Check sheet for the modelled part. Datum: model origin and axes. Units: mm. Round coordinates to 2 decimals unless told otherwise and drop trailing zeros. Write each loop counter-clockwise with the first axis right and the second up, starting at its lowest first coordinate (ties: lowest second). Pieces come first, ordered by that corner, then holes.
Item 1: Material ranges on line 1 along X through (y, z) = (42, 2.7); line 2 along X through (y, z) = (36, 0.9); line 3 along Y through (x, z) = (-52, 0.85), recorded low to high.
Item 2: Section check D-D, the plane z = 2.25. State how many separate pieces and enclosed holes the cut face has, plus the area to 3 significant figures.
Item 3: Section check C-C, the plane x = -11.5. Record the cut outline in (y, z), plus the area to 3 significant figures.
Item 4: Section check B-B, the plane y = 12. Record the cut outline in (x, z).
Item 5: Section check A-A, the plane y = 64. Record the cut outline in (x, z).
Item 6: Depth check by flat-ended pin: pin 1 (1.5 mm diameter, centred on y = 37, z = 1.5, fed in from +X). Enter the tip coordinate at first touch or a pass-through.
from build123d import *

# Parameters (mm, degrees)
F1_DEPTH = 3


with BuildPart() as f1:
    # F0 (on Top) → F1 (new body)
    with BuildSketch(Plane.XY):
        with BuildLine():
            Line((0, 20), (-26.666667, 20))
            ThreePointArc((-26.666667, 20), (-29.828944, 20.513167), (-32.666667, 22))
            Line((-32.666667, 22), (-30, 20))
            Line((-30, 20), (-30, 0.57191))
            ThreePointArc((-30, 0.57191), (-28.357686, 0.144014), (-26.666667, 0))
            Line((-26.666667, 0), (0, 0))
            Line((0, 0), (0, 10))
            Line((0, 10), (0, 20))
        make_face()
        with BuildLine():
            Line((26.666667, 20), (0, 20))
            Line((0, 20), (0, 10))
            Line((0, 10), (0, 0))
            Line((0, 0), (26.666667, 0))
            ThreePointArc((26.666667, 0), (28.357686, 0.144014), (30, 0.57191))
            Line((30, 0.57191), (30, 20))
            Line((30, 20), (32.666667, 22))
            ThreePointArc((32.666667, 22), (29.828944, 20.513167), (26.666667, 20))
        make_face()
        with BuildLine():
            Line((-30, 20), (-32.666667, 22))
            Line((-32.666667, 22), (-70.117305, 50.087979))
            Line((-70.117305, 50.087979), (-71.717305, 51.287979))
            Line((-71.717305, 51.287979), (-76.11797, 54.588477))
            ThreePointArc((-76.11797, 54.588477), (-78.558883, 57.226483), (-79.909473, 60.557104))
            ThreePointArc((-79.909473, 60.557104), (-104.817576, 66.113182), (-92.509473, 43.757104))
            ThreePointArc((-92.509473, 43.757104), (-88.933911, 43.393113), (-85.71797, 41.788477))
            Line((-85.71797, 41.788477), (-39.6, 7.2))
            Line((-39.6, 7.2), (-32.666667, 2))
            ThreePointArc((-32.666667, 2), (-31.387645, 1.184538), (-30, 0.57191))
            Line((-30, 0.57191), (-30, 20))
        make_face()
        Polygon((-64.226276, 29.419657), (-60.626276, 34.219657), (-56.226276, 23.419657), align=None, mode=Mode.SUBTRACT)
        Polygon((-74.7174, 37.28805), (-63.1174, 36.08805), (-66.7174, 31.28805), align=None, mode=Mode.SUBTRACT)
        Polygon((-50.3174, 31.488), (-53.9174, 26.688), (-58.3174, 37.488), align=None, mode=Mode.SUBTRACT)
        Polygon((-53.9174, 21.688), (-42.3174, 20.488), (-45.9174, 15.688), align=None, mode=Mode.SUBTRACT)
        Polygon((-39.9174, 23.688), (-51.5174, 24.888), (-47.9174, 29.688), align=None, mode=Mode.SUBTRACT)
        Polygon((-77.026276, 39.019707), (-85.026276, 45.019707), (-81.426276, 49.819707), align=None, mode=Mode.SUBTRACT)
        Polygon((-60.7174, 39.28805), (-72.3174, 40.48805), (-68.7174, 45.28805), align=None, mode=Mode.SUBTRACT)
        Polygon((-71.1174, 47.08805), (-74.7174, 42.28805), (-79.1174, 53.08805), align=None, mode=Mode.SUBTRACT)
        with BuildLine():
            ThreePointArc((-92.803023, 58.984095), (-92.361383, 58.454915), (-92.203023, 57.784095))
            ThreePointArc((-92.203023, 57.784095), (-92.279998, 57.309753), (-92.503023, 56.884095))
            ThreePointArc((-92.503023, 56.884095), (-93.490891, 56.299171), (-94.603023, 56.584095))
            ThreePointArc((-94.603023, 56.584095), (-95.187948, 57.571963), (-94.903023, 58.684095))
            ThreePointArc((-94.903023, 58.684095), (-93.915155, 59.269019), (-92.803023, 58.984095))
        make_face(mode=Mode.SUBTRACT)
        with BuildLine():
            Line((70.117305, 50.087979), (32.666667, 22))
            Line((32.666667, 22), (30, 20))
            Line((30, 20), (30, 0.57191))
            ThreePointArc((30, 0.57191), (31.387645, 1.184538), (32.666667, 2))
            Line((32.666667, 2), (39.6, 7.2))
            Line((39.6, 7.2), (85.71797, 41.788477))
            ThreePointArc((85.71797, 41.788477), (88.933911, 43.393113), (92.509473, 43.757104))
            ThreePointArc((92.509473, 43.757104), (104.817576, 66.113182), (79.909473, 60.557104))
            ThreePointArc((79.909473, 60.557104), (78.558883, 57.226483), (76.11797, 54.588477))
            Line((76.11797, 54.588477), (71.717305, 51.287979))
            Line((71.717305, 51.287979), (70.117305, 50.087979))
        make_face()
        Polygon((42.3174, 20.488), (53.9174, 21.688), (45.9174, 15.688), align=None, mode=Mode.SUBTRACT)
        Polygon((47.9174, 29.688), (51.5174, 24.888), (39.9174, 23.688), align=None, mode=Mode.SUBTRACT)
        Polygon((60.626276, 34.219657), (64.226276, 29.419657), (56.226276, 23.419657), align=None, mode=Mode.SUBTRACT)
        Polygon((58.3174, 37.488), (53.9174, 26.688), (50.3174, 31.488), align=None, mode=Mode.SUBTRACT)
        Polygon((74.7174, 37.28805), (66.7174, 31.28805), (63.1174, 36.08805), align=None, mode=Mode.SUBTRACT)
        Polygon((68.7174, 45.28805), (72.3174, 40.48805), (60.7174, 39.28805), align=None, mode=Mode.SUBTRACT)
        Polygon((81.426276, 49.819707), (85.026276, 45.019707), (77.026276, 39.019707), align=None, mode=Mode.SUBTRACT)
        Polygon((79.1174, 53.08805), (74.7174, 42.28805), (71.1174, 47.08805), align=None, mode=Mode.SUBTRACT)
        with BuildLine():
            ThreePointArc((94.903023, 58.684095), (95.126048, 58.258437), (95.203023, 57.784095))
            ThreePointArc((95.203023, 57.784095), (95.044664, 57.113275), (94.603023, 56.584095))
            ThreePointArc((94.603023, 56.584095), (93.490891, 56.299171), (92.503023, 56.884095))
            ThreePointArc((92.503023, 56.884095), (92.218099, 57.996227), (92.803023, 58.984095))
            ThreePointArc((92.803023, 58.984095), (93.915155, 59.269019), (94.903023, 58.684095))
        make_face(mode=Mode.SUBTRACT)
    extrude(amount=F1_DEPTH)


solid = f1.part
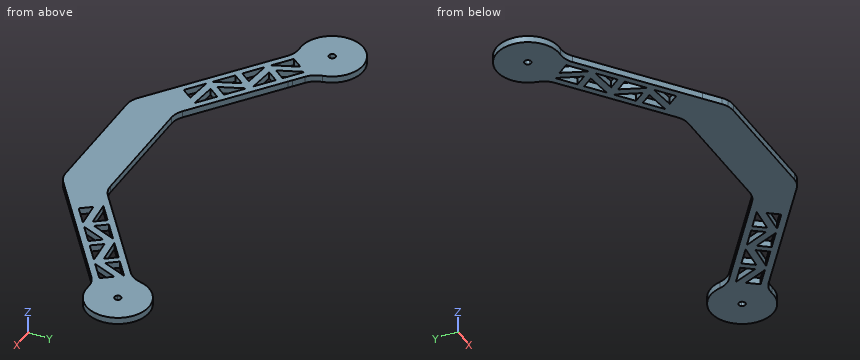
Values found:
1. line 1: x = -86.01 to -81, -78.24 to -71.18, -64.33 to -59.33, 59.33 to 64.33, 71.18 to 78.24, 81 to 86.01
1. line 2: x = -78 to -73, -63.18 to -57.71, -56.33 to -51.33, 51.33 to 56.33, 57.71 to 63.18, 73 to 78
1. line 3: y = 16.5 to 20.25, 21.49 to 29.24, 32.75 to 36.5
2. separate pieces: 1
2. enclosed holes: 18
2. area: 4,070 mm2
3. outline: (0, 0) - (20, 0) - (20, 3) - (0, 3) - close
3. area: 60.0 mm2
4. outline: (-46, 0) - (46, 0) - (46, 3) - (-46, 3) - close
5. outline: (-106.13, 0) - (-81.11, 0) - (-81.11, 3) - (-106.13, 3) - close; (81.11, 0) - (106.13, 0) - (106.13, 3) - (81.11, 3) - close
6. pin 1: stops at x = 80.33
